```python
from build123d import *

# Parameters (mm, degrees)
BOSS_EXTRUDE1_DEPTH = 23
SKETCH1_4_W         = 13.1
SKETCH1_4_H         = 9.8
CUT_EXTRUDE1_DEPTH  = 9
CHAMFER4_SIZE       = 10
CHAMFER6_SIZE       = 0.4
CUT_EXTRUDE5_DEPTH  = 43.713463919
FILLET1_R           = 0.4
CHAMFER7_SIZE       = 0.4


with BuildPart() as part:
    # Sketch1 → Boss-Extrude1 (new body)
    with BuildSketch(Plane.XY):
        with BuildLine():
            Line((-27, 6.1), (-15, 6.1))
            Line((-15, 6.1), (-15, 13))
            ThreePointArc((-15, 13), (-14.414213562, 14.414213562), (-13, 15))
            Line((-13, 15), (-6.55, 15))
            Line((-6.55, 15), (-6.55, 20.1))
            Line((-6.55, 20.1), (6.55, 20.1))
            Line((6.55, 20.1), (6.55, 15))
            Line((6.55, 15), (13, 15))
            ThreePointArc((13, 15), (14.414213562, 14.414213562), (15, 13))
            Line((15, 13), (15, 6.1))
            Line((15, 6.1), (27, 6.1))
            Line((27, 6.1), (27, 35))
            Line((27, 35), (6.55, 35))
            Line((6.55, 35), (6.55, 29.9))
            Line((6.55, 29.9), (-6.55, 29.9))
            Line((-6.55, 29.9), (-6.55, 35))
            Line((-6.55, 35), (-27, 35))
            Line((-27, 35), (-27, 6.1))
        make_face()
    extrude(amount=BOSS_EXTRUDE1_DEPTH)

    # Sketch1<4> → Cut-Extrude1 (cut)
    with BuildSketch(Plane.XY):
        with Locations((0, 25)):
            Rectangle(SKETCH1_4_W, SKETCH1_4_H)
    extrude(amount=CUT_EXTRUDE1_DEPTH, mode=Mode.SUBTRACT)

    # Chamfer4
    chamfer4_edges = [part.edges().sort_by_distance(p)[0] for p in [
        (-27, 35, 11.5),
        (27, 35, 11.5),
    ]]
    chamfer(chamfer4_edges, length=CHAMFER4_SIZE)

    # Chamfer6
    chamfer6_edges = [part.edges().sort_by_distance(p)[0] for p in [
        (17, 35, 11.5),
        (27, 25, 11.5),
        (-27, 25, 11.5),
        (-17, 35, 11.5),
    ]]
    chamfer(chamfer6_edges, length=CHAMFER6_SIZE)

    # Sketch6 → Cut-Extrude5 (cut, through all)
    with BuildSketch(Plane(origin=(0, 29.9, 0), x_dir=(1, 0, 0), z_dir=(0, 1, 0))):
        with BuildLine():
            ThreePointArc((1.75, -16.5), (1.237436867, -15.262563133), (0, -14.75))
            Line((0, -14.75), (0, -18.25))
            ThreePointArc((0, -18.25), (1.237436867, -17.737436867), (1.75, -16.5))
        make_face()
        with BuildLine():
            Line((0, -18.25), (0, -14.75))
            ThreePointArc((0, -14.75), (-1.75, -16.5), (0, -18.25))
        make_face()
    extrude(amount=-CUT_EXTRUDE5_DEPTH, mode=Mode.SUBTRACT)

    # Fillet1
    fillet1_edges = [part.edges().sort_by_distance(p)[0] for p in [
        (0, 29.9, 14.75),
    ]]
    fillet(fillet1_edges, radius=FILLET1_R)

    # Chamfer7
    chamfer7_edges = [part.edges().sort_by_distance(p)[0] for p in [
        (15, 9.55, 23),
        (16.941421356, 34.858578644, 0),
        (21, 6.1, 23),
        (27, 15.35, 23),
        (9.775, 15, 0),
        (6.55, 25, 0),
        (-6.55, 25, 0),
        (-9.775, 15, 0),
        (-14.414213562, 14.414213562, 0),
        (-15, 9.55, 0),
        (-21, 6.1, 0),
        (-11.575, 35, 0),
        (27, 15.35, 0),
        (21, 6.1, 0),
        (15, 9.55, 0),
        (14.414213562, 14.414213562, 0),
        (6.55, 32.45, 23),
        (6.55, 15, 11.5),
        (6.55, 20.1, 16),
        (-6.55, 20.1, 16),
        (-6.55, 15, 11.5),
        (-15, 6.1, 11.5),
        (-27, 6.1, 11.5),
        (-6.55, 35, 11.5),
        (-6.55, 29.9, 16),
        (6.55, 29.9, 16),
        (6.55, 35, 11.5),
        (27, 6.1, 11.5),
        (15, 6.1, 11.5),
        (0, 29.9, 23),
        (-6.55, 32.45, 23),
        (-11.575, 35, 23),
        (14.414213562, 14.414213562, 23),
        (-21, 6.1, 23),
        (0, 29.9, 9),
        (6.55, 25, 9),
        (-6.55, 25, 9),
        (0, 20.1, 9),
        (-15, 9.55, 23),
        (-14.414213562, 14.414213562, 23),
        (-9.775, 15, 23),
        (-6.55, 17.55, 23),
        (0, 20.1, 23),
        (-27, 15.35, 23),
        (-27, 15.35, 0),
        (6.55, 17.55, 23),
        (-22, 30, 0),
        (-16.941421356, 34.858578644, 0),
        (-26.858578644, 24.941421356, 0),
        (-22, 30, 23),
        (22, 30, 23),
        (9.775, 15, 23),
        (11.575, 35, 23),
        (26.858578644, 24.941421356, 23),
        (16.941421356, 34.858578644, 23),
        (-16.941421356, 34.858578644, 23),
        (-26.858578644, 24.941421356, 23),
        (11.575, 35, 0),
        (22, 30, 0),
        (26.858578644, 24.941421356, 0),
    ]]
    chamfer(chamfer7_edges, length=CHAMFER7_SIZE)


solid = part.part
```
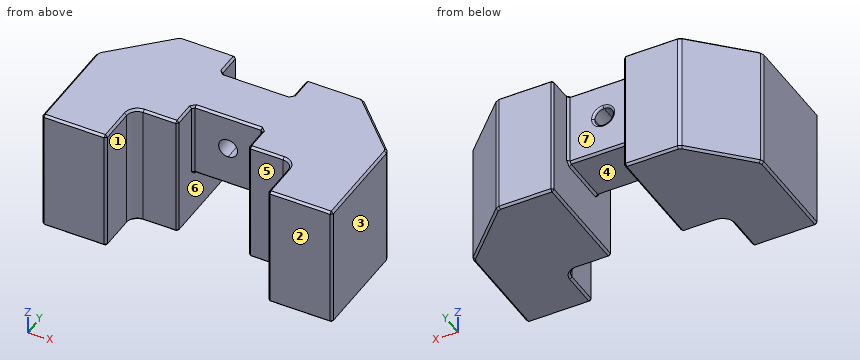
Here's how the part is built. I have some questions about the finished solid (model axes, mm). Face numbers are marked on the shaded views. A direction names the side the tool comes from. Coordinates: 2 decimals unless noted, no trailing zeros. Order: outer loops, then holes, each group sorted by start corner. A loop starts at its lowest first (then second) coordinate and runs counter-clockwise, first axis right, second up. Notation, with made-up numbers: (25, 89.25) - (50, 89.25) arc R25 ccw to (50, 111.25) - close; hole circle Ø3 at (72, 59.25). An arc over 180 degrees is marked (long way). One line per question, with ' | ' between items. Start each with the question number.
1. I'm going to push flat-ended pins straight in: pin 1 Ø8 at (x, z) = (10, 11) entering from -Y; pin 2 Ø3 at (x, z) = (9, 11.5) entering from -Y; pin 3 Ø4.5 at (x, y) = (-2, 24) entering from -Z. Where does each tip first touch, or does it pass through?
2. If we mould it in two halves opening along X, with no side actions, what happens to the marked faces 1, 2 and 3? For each: released by +X, released by -X, zero draft, split by the parting line, or undercut.
3. Please list where these lines run through material, in increasing order: line 1 along X through (y, z) = (11, 6); line 2 along X through (y, z) = (19.25, 7.5); line 3 along Z through (x, y) = (0, 27). Write a range as [from, to].
4. If we section it at D-D (y = 18): Write out the boundary of the cut face in (x, z), and give its area (3 significant figures).
5. If we section it at A-A (y = 12.25): Write out the boundary of the cut face in (x, z), and give its area (3 significant figures).
6. Which directions (+Z, -Z, +X, -X, +Y, -Y) give clear straight access to the entire face, cutting with the end or side of a thin tool? Please do the marked faces 4, 5, 6 and 7.
7. If we section it at C-C (x = 8): Write out the boundary of the cut face in (y, z).
8. If we section it at B-B (z = 6): Write out the boundary of the cut face in (x, y), and give its area (3 significant figures).
Model answer:
1) pin 1: stops at y = 14.73 | pin 2: stops at y = 15 | pin 3: stops at z = 9
2) face 1: undercut | face 2: zero draft | face 3: released by +X
3) line 1: x = [-27, -15], [15, 27] | line 2: x = [-27, -6.55], [6.55, 27] | line 3: z = [9, 14.75], [18.25, 23]
4) outline: (-27, 0.4) - (-26.6, 0) - (-6.95, 0) - (-6.55, 0.4) - (-6.55, 22.6) - (-6.95, 23) - (-26.6, 23) - (-27, 22.6) - close; (6.55, 0.4) - (6.95, 0) - (26.6, 0) - (27, 0.4) - (27, 22.6) - (26.6, 23) - (6.95, 23) - (6.55, 22.6) - close | area: 940 mm²
5) outline: (-27, 0.4) - (-26.6, 0) - (-15.4, 0) - (-15, 0.4) - (-15, 22.6) - (-15.4, 23) - (-26.6, 23) - (-27, 22.6) - close; (15, 0.4) - (15.4, 0) - (26.6, 0) - (27, 0.4) - (27, 22.6) - (26.6, 23) - (15.4, 23) - (15, 22.6) - close | area: 551 mm²
6) face 4: -Z, +Y, -Y | face 5: +Z, -Z, -Y | face 6: -Z | face 7: +Z, -Z, +Y
7) outline: (15, 0.4) - (15.4, 0) - (34.6, 0) - (35, 0.4) - (35, 22.6) - (34.6, 23) - (15.4, 23) - (15, 22.6) - close
8) outline: (-27, 6.5) - (-26.6, 6.1) - (-15.4, 6.1) - (-15, 6.5) - (-15, 13) arc R2 cw to (-13, 15) - (-6.95, 15) - (-6.55, 15.4) - (-6.55, 34.6) - (-6.95, 35) - (-16.6, 35) - (-17.28, 34.72) - (-26.72, 25.28) - (-27, 24.6) - close; (6.55, 15.4) - (6.95, 15) - (13, 15) arc R2 cw to (15, 13) - (15, 6.5) - (15.4, 6.1) - (26.6, 6.1) - (27, 6.5) - (27, 24.6) - (26.72, 25.28) - (17.28, 34.72) - (16.6, 35) - (6.95, 35) - (6.55, 34.6) - close | area: 932 mm²
